Read the model definition and answer for the solid it produces. Units are mm, in the model's axes. A direction names the side the tool comes from. Coordinates: 2 decimals unless noted, no trailing zeros. Write each loop counter-clockwise with the first axis right and the second up, starting at its lowest first coordinate (ties: lowest second). Pieces come first, ordered by that corner, then holes. Notation, with made-up numbers: (-23.5, -37.5) -> (35.5, -37.5) arc R18 ccw to (35.5, -21.5) -> close; hole circle Ø1 at (45, 76). An arc over 180 degrees is marked (long way). Use CSV: the item, a comma, the result in double quotes.
from build123d import *

# Parameters (mm, degrees)
BOSS_EXTRUDE1_START       = 3
SKETCH1_R                 = 27.5
SKETCH1_R_2               = 14
BOSS_EXTRUDE1_DEPTH       = 18
BOSS_EXTRUDE2_START       = 18
SKETCH1_3_R               = 14
BOSS_EXTRUDE2_DEPTH       = 3
BOSS_EXTRUDE3_START       = 9
SKETCH1_4_R               = 14
SKETCH1_4_R_2             = 13
BOSS_EXTRUDE3_DEPTH       = 9
CUT_EXTRUDE1_REACH        = 44.854
SKETCH2_R                 = 2.1
SKETCH2_3_R               = 3.75
SKETCH2_3_R_2             = 2.1
CUT_EXTRUDE2_DEPTH        = 4.5
CHAMFER1_SIZE             = 0.5
BOSS_EXTRUDE4_START       = 3
BOSS_EXTRUDE4_OUTLINE_R   = 14
BOSS_EXTRUDE4_OUTLINE_R_2 = 13
BOSS_EXTRUDE4_DEPTH       = 4.84
BOSS_EXTRUDE5_START       = 1
SKETCH3_R                 = 13
BOSS_EXTRUDE5_DEPTH       = 1
SKETCH4_R                 = 35
CUT_EXTRUDE3_DEPTH        = 3.5
CUT_EXTRUDE5_REACH        = 42.283
SKETCH5_R                 = 6
FILLET1_R                 = 7


# Read off the part's stored shape, not the designer's step: Boss-Extrude4
with BuildPart() as part:
    # Sketch1 → Boss-Extrude1 (new body)
    with BuildSketch(Plane(origin=(0, 0, 0), x_dir=(1, 0, 0), z_dir=(0, 1, 0)).offset(BOSS_EXTRUDE1_START)):
        with Locations(Location((0, 0, 0), (0, 0, 270))):
            Circle(SKETCH1_R)
        with Locations(Location((0, 0, 0), (0, 0, 270))):
            Circle(SKETCH1_R_2, mode=Mode.SUBTRACT)
    extrude(amount=BOSS_EXTRUDE1_DEPTH)

    # Sketch1<3> → Boss-Extrude2 (add)
    with BuildSketch(Plane(origin=(0, 0, 0), x_dir=(1, 0, 0), z_dir=(0, 1, 0)).offset(BOSS_EXTRUDE2_START)):
        with Locations(Location((0, 0, 0), (0, 0, 270))):
            Circle(SKETCH1_3_R)
    extrude(amount=BOSS_EXTRUDE2_DEPTH)

    # Sketch1<4> → Boss-Extrude3 (add)
    with BuildSketch(Plane(origin=(0, 0, 0), x_dir=(1, 0, 0), z_dir=(0, 1, 0)).offset(BOSS_EXTRUDE3_START)):
        with Locations(Location((0, 0, 0), (0, 0, 270))):
            Circle(SKETCH1_4_R)
        with Locations(Location((0, 0, 0), (0, 0, 270))):
            Circle(SKETCH1_4_R_2, mode=Mode.SUBTRACT)
    extrude(amount=BOSS_EXTRUDE3_DEPTH)

    # Sketch2 → Cut-Extrude1 (cut, up to next)
    with BuildSketch(Plane(origin=(0, 21, 0), x_dir=(1, 0, 0), z_dir=(0, 1, 0)), mode=Mode.PRIVATE) as cut_extrude1_sk1:
        with Locations(Location((0, -20, 0), (0, 0, 270))):
            Circle(SKETCH2_R)
    cut_extrude1_tool1 = extrude(cut_extrude1_sk1.sketch, amount=-CUT_EXTRUDE1_REACH, mode=Mode.PRIVATE) & part.part
    # Sketch2 → Cut-Extrude1 (cut, up to next)
    with BuildSketch(Plane(origin=(0, 21, 0), x_dir=(1, 0, 0), z_dir=(0, 1, 0)), mode=Mode.PRIVATE) as cut_extrude1_sk2:
        with Locations(Location((-20, 0, 0), (0, 0, 270))):
            Circle(SKETCH2_R)
    cut_extrude1_tool2 = extrude(cut_extrude1_sk2.sketch, amount=-CUT_EXTRUDE1_REACH, mode=Mode.PRIVATE) & part.part
    # Sketch2 → Cut-Extrude1 (cut, up to next)
    with BuildSketch(Plane(origin=(0, 21, 0), x_dir=(1, 0, 0), z_dir=(0, 1, 0)), mode=Mode.PRIVATE) as cut_extrude1_sk3:
        with Locations(Location((20, 0, 0), (0, 0, 270))):
            Circle(SKETCH2_R)
    cut_extrude1_tool3 = extrude(cut_extrude1_sk3.sketch, amount=-CUT_EXTRUDE1_REACH, mode=Mode.PRIVATE) & part.part
    # Sketch2 → Cut-Extrude1 (cut, up to next)
    with BuildSketch(Plane(origin=(0, 21, 0), x_dir=(1, 0, 0), z_dir=(0, 1, 0)), mode=Mode.PRIVATE) as cut_extrude1_sk4:
        with Locations(Location((0, 20, 0), (0, 0, 270))):
            Circle(SKETCH2_R)
    cut_extrude1_tool4 = extrude(cut_extrude1_sk4.sketch, amount=-CUT_EXTRUDE1_REACH, mode=Mode.PRIVATE) & part.part
    add(cut_extrude1_tool1.solids().sort_by_distance((0, 21, 20))[0], mode=Mode.SUBTRACT)
    add(cut_extrude1_tool2.solids().sort_by_distance((-20, 21, 0))[0], mode=Mode.SUBTRACT)
    add(cut_extrude1_tool3.solids().sort_by_distance((20, 21, 0))[0], mode=Mode.SUBTRACT)
    add(cut_extrude1_tool4.solids().sort_by_distance((0, 21, -20))[0], mode=Mode.SUBTRACT)

    # Sketch2<3> → Cut-Extrude2 (cut)
    # profile 1 of 4: a face of its own
    with BuildSketch(Plane(origin=(0, 21, 0), x_dir=(1, 0, 0), z_dir=(0, 1, 0))):
        with Locations(Location((0, -20, 0), (0, 0, 270))):
            Circle(SKETCH2_3_R)
        with Locations(Location((0, -20, 0), (0, 0, 270))):
            Circle(SKETCH2_3_R_2, mode=Mode.SUBTRACT)
    # profile 2 of 4: a face of its own
    with BuildSketch(Plane(origin=(0, 21, 0), x_dir=(1, 0, 0), z_dir=(0, 1, 0))):
        with Locations(Location((-20, 0, 0), (0, 0, 270))):
            Circle(SKETCH2_3_R)
        with Locations(Location((-20, 0, 0), (0, 0, 270))):
            Circle(SKETCH2_3_R_2, mode=Mode.SUBTRACT)
    # profile 3 of 4: a face of its own
    with BuildSketch(Plane(origin=(0, 21, 0), x_dir=(1, 0, 0), z_dir=(0, 1, 0))):
        with Locations(Location((0, 20, 0), (0, 0, 270))):
            Circle(SKETCH2_3_R)
        with Locations(Location((0, 20, 0), (0, 0, 270))):
            Circle(SKETCH2_3_R_2, mode=Mode.SUBTRACT)
    # profile 4 of 4: a face of its own
    with BuildSketch(Plane(origin=(0, 21, 0), x_dir=(1, 0, 0), z_dir=(0, 1, 0))):
        with Locations(Location((20, 0, 0), (0, 0, 270))):
            Circle(SKETCH2_3_R)
        with Locations(Location((20, 0, 0), (0, 0, 270))):
            Circle(SKETCH2_3_R_2, mode=Mode.SUBTRACT)
    extrude(amount=-CUT_EXTRUDE2_DEPTH, mode=Mode.SUBTRACT)

    # Chamfer1
    chamfer1_edges = [part.edges().sort_by_distance(p)[0] for p in [
        (0, 16.5, 17.9),
        (-20, 16.5, -2.1),
        (0, 16.5, -22.1),
        (20, 16.5, -2.1),
    ]]
    chamfer(chamfer1_edges, length=CHAMFER1_SIZE)

    # Boss-Extrude4 outline → Boss-Extrude4 (add)
    with BuildSketch(Plane(origin=(0, 0, 0), x_dir=(1, 0, 0), z_dir=(0, 1, 0)).offset(BOSS_EXTRUDE4_START)):
        Circle(BOSS_EXTRUDE4_OUTLINE_R)
        Circle(BOSS_EXTRUDE4_OUTLINE_R_2, mode=Mode.SUBTRACT)
    extrude(amount=BOSS_EXTRUDE4_DEPTH)

    # Sketch3 → Boss-Extrude5 (add)
    with BuildSketch(Plane.XZ.offset(-18).offset(BOSS_EXTRUDE5_START)):
        with Locations(Location((0, 0, 0), (0, 0, 270))):
            Circle(SKETCH3_R)
    extrude(amount=-BOSS_EXTRUDE5_DEPTH)

    # Sketch4 → Cut-Extrude3 (cut)
    with BuildSketch(Plane.XZ.offset(-3)):
        Circle(SKETCH4_R)
    extrude(amount=-CUT_EXTRUDE3_DEPTH, mode=Mode.SUBTRACT)

    # Sketch5 → Cut-Extrude5 (cut, up to next)
    with BuildSketch(Plane.XZ.offset(-17), mode=Mode.PRIVATE) as cut_extrude5_sk1:
        with Locations(Location((0, 0, 0), (0, 0, 270))):
            Circle(SKETCH5_R)
    cut_extrude5_tool1 = extrude(cut_extrude5_sk1.sketch, amount=-CUT_EXTRUDE5_REACH, mode=Mode.PRIVATE) & part.part
    add(cut_extrude5_tool1.solids().sort_by_distance((0, 17, 0))[0], mode=Mode.SUBTRACT)

    # Fillet1
    # the kernel refuses this fillet: 7 mm, written as the material it takes off along each edge
    with BuildSketch(Plane(origin=(0, 21, 0), x_dir=(0, 0, 1), z_dir=(-1, 0, 0))) as fillet1_piece_1:
        with BuildLine():
            CenterArc((27.5 - FILLET1_R, -FILLET1_R), FILLET1_R, 0, 90)
            Line((27.5 - FILLET1_R, 0), (27.5, 0))
            Line((27.5, 0), (27.5, -FILLET1_R))
        make_face()
    revolve(axis=Axis((0, 21, 0), (0, 1, 0)), mode=Mode.SUBTRACT)


solid = part.part
1. A cutting plane is placed at B-B (z = 0). Give the number of separate pieces and of enclosed holes in the cut face, and give its area (3 significant figures).
Solutions:
separate pieces,"4"
enclosed holes,"0"
area,"303 mm^2"
2. A cutting plane is placed at A-A (y = 13). Give the vertices of the cut face in (x, z).
Solutions:
outline,"circle Ø55 at (0, 0); hole circle Ø4.2 at (-20, 0); hole circle Ø26 at (0, 0); hole circle Ø4.2 at (0, -20); hole circle Ø4.2 at (0, 20); hole circle Ø4.2 at (20, 0)"
3. Find the intervals of material crossed by line 1 along X through (y, z) = (6.85, 0); line 2 along X through (y, z) = (19.95, 0); line 3 along Z through (x, y) = (1, 14.25), in increasing order.
Solutions:
line 1,"x = -27.5 to -22.1, -17.9 to -13, 13 to 17.9, 22.1 to 27.5"
line 2,"x = -24.19 to -23.75, -16.25 to -6, 6 to 16.25, 23.75 to 24.19"
line 3,"z = -27.48 to -21.85, -18.15 to -12.96, 12.96 to 18.15, 21.85 to 27.48"
4. Each of these flat-tipped pins is pushed along its axis until it touches: pin 1 Ø4 at (x, z) = (0, -20) entering from -Y; pin 2 Ø4 at (x, z) = (-19.5, -1) entering from +Y; pin 3 Ø3 at (x, y) = (-3.5, 14) entering from +Z; pin 4 Ø5 at (y, z) = (11.5, 6) entering from -X. Where does it stop, or does it pass through?
Solutions:
pin 1,"passes through"
pin 2,"stops at y = 16.5"
pin 3,"stops at z = 27.43"
pin 4,"stops at x = -27.28"
5. For a pull along Z with two mould halves and no side action, classify faces 1 (the cylindrical face through (21.77, 11.32, 1.13)), 2 (the cylindrical face through (-24.397, 10.198, 12.69)), 3 (the flat face through (5, 21, -5)) as pulls with the +Z half, pulls with the -Z half, needs draft (parallel to the pull), parting line crosses it, or undercut.
Solutions:
face 1,"undercut"
face 2,"parting line crosses it"
face 3,"needs draft"
6. A cutting plane is placed at C-C (y = 18). Give the vertices of the cut face in (x, z).
Solutions:
outline,"circle Ø52.49 at (0, 0); hole circle Ø7.5 at (-20, 0); hole circle Ø12 at (0, 0); hole circle Ø7.5 at (0, -20); hole circle Ø7.5 at (0, 20); hole circle Ø7.5 at (20, 0)"
7. A tool of negligible diameter and unlimited length cuts with its end or side. For faces 4 (the flat face through (-3, 17, -6)), 5 (the cylindrical face through (-5.362, 8.412, 12.932)), 6 (the cylindrical face through (-1.436, 18.782, -16.536)), 7 (the cylindrical face through (-18.23, 11.32, 1.13)), 8 (the flat face through (12, 6.5, -6)), from which of +Z, -Z, +X, -X, +Y, -Y can it reach the whole face along a straight path? Write none if from no direction.
Solutions:
face 4,"-Y"
face 5,"none"
face 6,"+Y"
face 7,"+Y, -Y"
face 8,"+Z, -Z, +X, -X, -Y"
